Autodesk Inventor part; units mm, degrees
ref_plane "YZ Plane" through (0, 0, 0) normal (1, 0, 0) x (0, 1, 0)
ref_plane "XZ Plane" through (0, 0, 0) normal (0, 1, 0) x (-1, 0, 0)
ref_plane "XY Plane" through (0, 0, 0) normal (0, 0, 1) x (1, 0, 0)
sketch "スケッチ1" plane through (0, 0, 0) normal (0, 1, 0) x (-1, 0, 0)
  line L0 (-7.5, -7.5) -> (7.5, -7.5)
  line L1 (7.5, -7.5) -> (7.5, 7.5)
  line L2 (7.5, 7.5) -> (-7.5, 7.5)
  line L3 (-7.5, 7.5) -> (-7.5, -7.5)
  line L4 (-7.5, -7.5) -> (7.5, 7.5) construction
  line L5 (7.5, -7.5) -> (-7.5, 7.5) construction
  line L6 (6.5, 6.5) -> (6.5, -6.5)
  line L7 (6.5, -6.5) -> (-6.5, -6.5)
  line L8 (-6.5, -6.5) -> (-6.5, 6.5)
  line L9 (-6.5, 6.5) -> (6.5, 6.5)
  point P0 (0, 0)
  dimension "d0" = 15
  dimension "d1" = 15
extrude "押し出し1" add sketch "スケッチ1" along normal mid plane 200
sketch "スケッチ3" plane through (-7.5, -100, 7.5) normal (-1, 0, 0) x (0, 0, 1)
  line L0 (-7.5, 177.5) -> (-7.5, 22.5)
  line L1 (0, 0) -> (-15, 0)
  point P0 (-7.5, 100)
  point P1 (-7.5, 100)
  dimension "d20" = 22.5
hole "穴1" at (-7.5, 77.5, 0) at (-7.5, -77.5, 0) direction (1, 0, 0) diameter 3.2 end through all
sketch "スケッチ4" plane through (7.5, 100, -7.5) normal (0, 0, -1) x (-1, 0, 0)
  line L0 (7.5, -7.5) -> (7.5, -192.5)
  line L1 (15, -200) -> (0, -200)
  point P0 (7.5, -100)
  point P1 (7.5, -100)
  dimension "d21" = 7.5
hole "穴2" at (0, 92.5, -7.5) at (0, -92.5, -7.5) direction (0, 0, 1) diameter 3.2 end through all
properties part number "回路角柱L200"
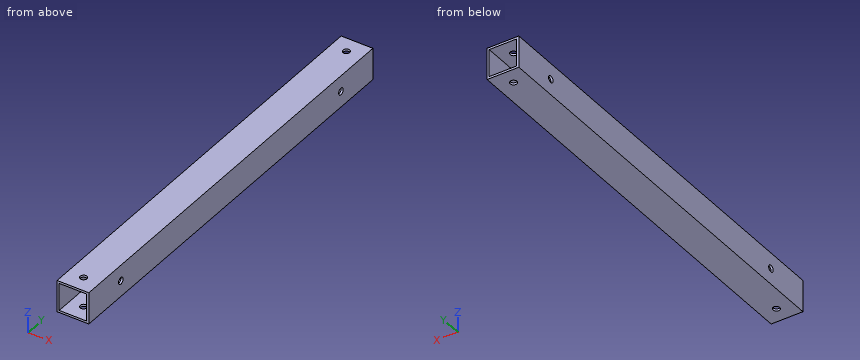
Geometry: final body of the model. Coordinates: model frame, mm. Round coordinates to 2 decimals unless told otherwise and drop trailing zeros. Order: outer loops, then holes, each group sorted by start corner. A loop starts at its lowest first (then second) coordinate and runs counter-clockwise, first axis right, second up. Notation, with made-up numbers: (-25, 31) -> (29, 31) arc R18 ccw to (29, 53) -> close; hole circle Ø3 at (81, -24.75). An arc over 180 degrees is marked (long way). Use one line per item in the form item = value.
(1) Section B-B on y = -66. Return loops of the section in (x, z), and give its area (3 significant figures).
Results list:
outline = (-7.5, -7.5) -> (7.5, -7.5) -> (7.5, 7.5) -> (-7.5, 7.5) -> close; hole (-6.5, -6.5) -> (6.5, -6.5) -> (6.5, 6.5) -> (-6.5, 6.5) -> close
area = 56.0 mm^2
(2) Ray query, probe 1 along Y at (x, z) = (-7, 0); probe 2 along Y at (x, z) = (0, 6.9); probe 3 along X at (y, z) = (-33, 2.25). Return the intervals inside material, ascending. Write a range as [from, to].
Results list:
probe_1 = [-100, -79.1], [-75.9, 75.9], [79.1, 100]
probe_2 = [-100, -94.1], [-90.9, 90.9], [94.1, 100]
probe_3 = [-7.5, -6.5], [6.5, 7.5]
(3) Section A-A on z = 3.25. Return loops of the section in (x, y).
Results list:
outline = (-7.5, -100) -> (-6.5, -100) -> (-6.5, 100) -> (-7.5, 100) -> close; (6.5, -100) -> (7.5, -100) -> (7.5, 100) -> (6.5, 100) -> close
